Could you check a few things on this drawing? It's one solid part, dimensions in mm from its lowest x, y, z. A direction names the side the tool comes from. Coordinates: 2 decimals unless noted, no trailing zeros. Write each loop counter-clockwise with the first axis right and the second up, starting at its lowest first coordinate (ties: lowest second). Pieces come first, ordered by that corner, then holes. Notation, with made-up numbers: (26.5, 17) - (41.5, 17) arc R27 cw to (41.5, 39) - close; hole circle Ø2 at (-21, 86.5). An arc over 180 degrees is marked (long way). Use one line per item in the form item = value. Start each with the question number.
(1) For pin 1 Ø3 at (y, z) = (20.5, 2.5) entering from +X; pin 2 Ø5 at (x, z) = (106.5, 12) entering from -Y; pin 3 Ø2 at (y, z) = (7, 16) entering from -X; pin 4 Ø18 at (x, y) = (219.2, 25) entering from -Z, each with a flat end and sliding along its axis, tell me the tip position at first contact or that it passes through.
(2) If we section it at A-A on y = 37.5: Give the number of separate pieces and of enclosed holes in the cut face, then the cut area to 3 significant figures.
(3) If we section it at D-D on x = 112: Please give me the cut outline in (y, z), then the cut area to 3 significant figures.
(4) If we section it at B-B on x = 208.5: Please give me the cut outline in (y, z) (1 decimal).
(5) If we section it at C-C on x = 53: Please give me the cut outline in (y, z), then the cut area to 3 significant figures.
(6) If I drill on probe 1 along X at (y, z) = (40.5, 1.25) (1 decimal); probe 2 along X at (y, z) = (26, 14.75); probe 3 along Z at (x, y) = (212.5, 45), over which ranges is the centre line in solid material (lowest first)? Write a range as from..to.
(7) On a 3-axis mill with a long thin cutter (end or side, diameter ignored), from which of +Z, -Z, +X, -X, +Y, -Y can I reach the whole of each face in a straight line? I mean the marked faces 1, 2, 3, 4 and 5. Say none if no direction works.
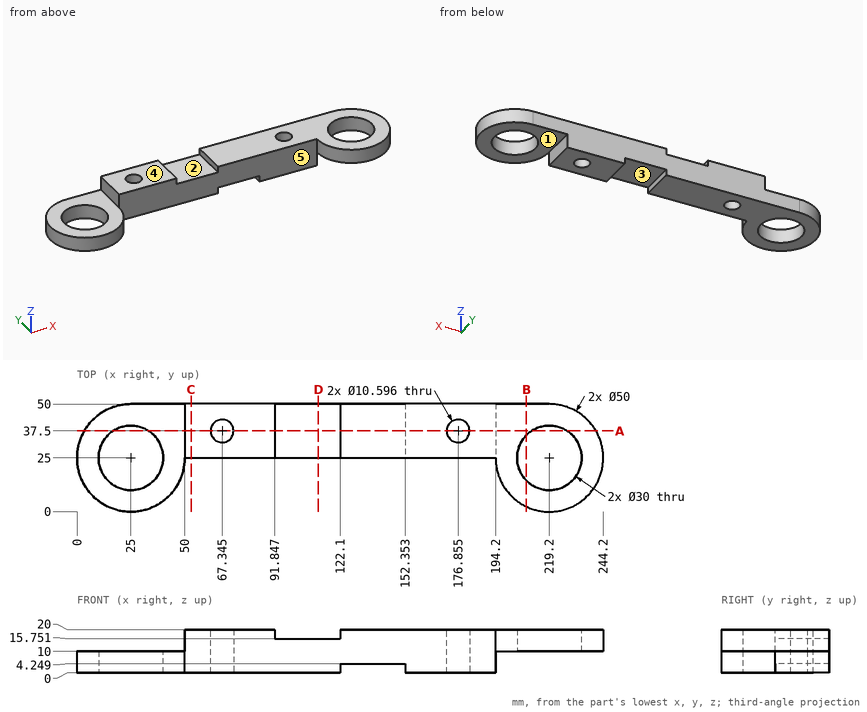
Reported:
q1.pin_1 = 49.82
q1.pin_2 = 25
q1.pin_3 = 200.87
q1.pin_4 = through
q2.separate_pieces = 5
q2.enclosed_holes = 0
q2.area = 2,800 mm2
q3.outline = (25, 0) - (50, 0) - (50, 15.75) - (25, 15.75) - close
q3.area = 394 mm2
q4.outline = (2.4, 10) - (14.5, 10) - (14.5, 20) - (2.4, 20) - close; (35.5, 10) - (50, 10) - (50, 20) - (35.5, 20) - close
q5.outline = (25, 0) - (50, 0) - (50, 20) - (25, 20) - close
q5.area = 500 mm2
q6.probe_1 = 5.4..63, 71.7..122.1, 152.4..172.5, 181.2..194.2
q6.probe_2 = 50..204.23, 234.17..244.18
q6.probe_3 = 10..20
q7.face_1 = -Z, +X, +Y, -Y
q7.face_2 = +Z, +Y, -Y
q7.face_3 = -Z, +Y, -Y
q7.face_4 = +Z, +X, -X, +Y, -Y
q7.face_5 = +Z, -Z, -Y
